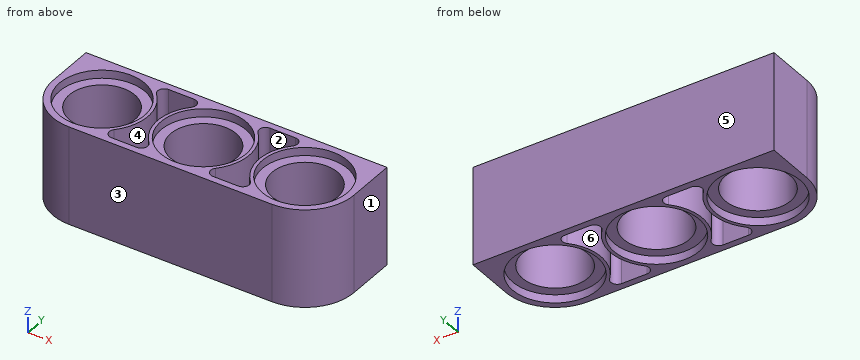
```python
from build123d import *

# Parameters (mm, degrees)
SKETCH1_R           = 3.302
SKETCH1_R_2         = 2.54
BOSS_EXTRUDE1_DEPTH = 3.81
SKETCH1_7_R         = 2.54
BOSS_EXTRUDE2_DEPTH = 3.81
SKETCH2_R           = 3.302
CUT_EXTRUDE1_DEPTH  = 0.635
BOSS_EXTRUDE3_DEPTH = 7.62


with BuildPart() as part:
    # Sketch1 → Boss-Extrude1 (new body)
    with BuildSketch(Plane.XY):
        with BuildLine():
            Line((3.937, -3.81), (7.874, -3.81))
            ThreePointArc((7.874, -3.81), (11.684, 0), (7.874, 3.81))
            Line((7.874, 3.81), (3.937, 3.81))
            Line((3.937, 3.81), (3.937, 3.302))
            Line((3.937, 3.302), (4.92278669, 3.302))
            ThreePointArc((4.92278669, 3.302), (5.389414486, 2.994804631), (5.291688354, 2.44475))
            ThreePointArc((5.291688354, 2.44475), (4.318, 0), (5.291688354, -2.44475))
            ThreePointArc((5.291688354, -2.44475), (5.389414486, -2.994804631), (4.92278669, -3.302))
            Line((4.92278669, -3.302), (3.937, -3.302))
            Line((3.937, -3.302), (3.937, -3.81))
        make_face()
        with Locations((7.874, 0)):
            Circle(SKETCH1_R, mode=Mode.SUBTRACT)
        with Locations((7.874, 0)):
            Circle(SKETCH1_R)
        with Locations(Location((7.874, 0, 0), (0, 0, 180))):
            Circle(SKETCH1_R_2, mode=Mode.SUBTRACT)
    extrude(amount=BOSS_EXTRUDE1_DEPTH)


with BuildPart() as body_2:
    # Sketch1_7 → Boss-Extrude2 (new body)
    with BuildSketch(Plane.XY):
        with BuildLine():
            Line((3.937, -3.81), (3.937, -3.302))
            Line((3.937, -3.302), (2.95121331, -3.302))
            ThreePointArc((2.95121331, -3.302), (2.484585514, -2.994804631), (2.582311646, -2.44475))
            ThreePointArc((2.582311646, -2.44475), (3.556, 0), (2.582311646, 2.44475))
            ThreePointArc((2.582311646, 2.44475), (2.484585514, 2.994804631), (2.95121331, 3.302))
            Line((2.95121331, 3.302), (3.937, 3.302))
            Line((3.937, 3.302), (3.937, 3.81))
            Line((3.937, 3.81), (-3.937, 3.81))
            Line((-3.937, 3.81), (-3.937, 3.302))
            Line((-3.937, 3.302), (-2.95121331, 3.302))
            ThreePointArc((-2.95121331, 3.302), (-2.484585514, 2.994804631), (-2.582311646, 2.44475))
            ThreePointArc((-2.582311646, 2.44475), (-3.556, 0), (-2.582311646, -2.44475))
            ThreePointArc((-2.582311646, -2.44475), (-2.484585514, -2.994804631), (-2.95121331, -3.302))
            Line((-2.95121331, -3.302), (-3.937, -3.302))
            Line((-3.937, -3.302), (-3.937, -3.81))
            Line((-3.937, -3.81), (3.937, -3.81))
        make_face()
        with Locations(Location((0, 0, 0), (0, 0, 180))):
            Circle(SKETCH1_7_R, mode=Mode.SUBTRACT)
    extrude(amount=BOSS_EXTRUDE2_DEPTH)


with BuildPart() as cut_extrude1_tool:
    # Sketch2 → Cut-Extrude1 (new body)
    with BuildSketch(Plane.XY):
        with Locations((7.874, 0)):
            Circle(SKETCH2_R)
        Circle(SKETCH2_R)
    extrude(amount=CUT_EXTRUDE1_DEPTH)


with BuildPart() as part_1:
    add(part.part)

    # Cut-Extrude1: cut by cut_extrude1_tool
    add(cut_extrude1_tool.part, mode=Mode.SUBTRACT)


with BuildPart() as body_2_1:
    add(body_2.part)

    # Cut-Extrude1: cut by cut_extrude1_tool
    add(cut_extrude1_tool.part, mode=Mode.SUBTRACT)


with BuildPart() as body_3:
    # Mirror2: mirrored copy
    add(part_1.part.mirror(Plane(origin=(0, 0, 0), x_dir=(0, 0, 1), z_dir=(1, 0, 0))))


with BuildPart() as part_2:
    add(part_1.part)

    # Combine1: union body 3, body 2
    add(body_3.part)
    add(body_2_1.part)

    # Mirror3: part across plane


with BuildPart() as part_3:
    add(part_2.part)
    add(part_2.part.mirror(Plane.XY.offset(3.81)))

    # Sketch3 → Boss-Extrude3 (add, through all)
    with BuildSketch(Plane.XY.offset(7.62)):
        with BuildLine():
            Line((7.874, 3.81), (11.684, 3.81))
            Line((11.684, 3.81), (11.684, 0))
            ThreePointArc((11.684, 0), (10.568076836, 2.694076836), (7.874, 3.81))
        make_face()
    boss_extrude3 = extrude(amount=-BOSS_EXTRUDE3_DEPTH)

    # Mirror4: Boss-Extrude3 across plane
    add(boss_extrude3.mirror(Plane(origin=(0, 0, 0), x_dir=(0, 0, 1), z_dir=(1, 0, 0))))


solid = part_3.part
```
Check sheet for the modelled part. Datum: model origin and axes. Units: mm. Face numbers are marked on the shaded views. A direction names the side the tool comes from. Coordinates: 2 decimals unless noted, no trailing zeros. Write each loop counter-clockwise with the first axis right and the second up, starting at its lowest first coordinate (ties: lowest second). Pieces come first, ordered by that corner, then holes. Notation, with made-up numbers: (83, -26.5) - (138, -26.5) arc R26 cw to (138, -10.5) - close; hole circle Ø8 at (78.25, 69.5). An arc over 180 degrees is marked (long way). One line per question, with ' | ' between items.
Item 1: Mould release check, pull along X, two halves, no side actions. Record for the marked faces 1, 2, 3 and 4: pulls with the +X half, pulls with the -X half, needs draft (parallel to the pull), parting line crosses it, or undercut.
Determined:
face 1: pulls with the +X half | face 2: undercut | face 3: needs draft | face 4: undercut
Item 2: Sectioned sample at A-A on z = 2.5. Record the boundary of the cut face in (x, y), plus the area to 3 significant figures.
Determined:
outline: (-11.68, 0) arc R3.81 ccw to (-7.87, -3.81) - (7.87, -3.81) arc R3.81 ccw to (11.68, 0) - (11.68, 3.81) - (-11.68, 3.81) - close; hole circle Ø5.08 at (-7.87, 0); hole (-5.29, -2.44) arc R0.51 ccw to (-4.92, -3.3) - (-2.95, -3.3) arc R0.51 ccw to (-2.58, -2.44) arc R3.56 cw to (-2.58, 2.44) arc R0.51 ccw to (-2.95, 3.3) - (-4.92, 3.3) arc R0.51 ccw to (-5.29, 2.44) arc R3.56 cw to start; hole circle Ø5.08 at (0, 0); hole (2.58, -2.44) arc R0.51 ccw to (2.95, -3.3) - (4.92, -3.3) arc R0.51 ccw to (5.29, -2.44) arc R3.56 cw to (5.29, 2.44) arc R0.51 ccw to (4.92, 3.3) - (2.95, 3.3) arc R0.51 ccw to (2.58, 2.44) arc R3.56 cw to start; hole circle Ø5.08 at (7.87, 0) | area: 87.9 mm2
Item 3: Sectioned sample at B-B on x = 0. Record the boundary of the cut face in (y, z) (3 decimals), plus the area to 3 significant figures.
Determined:
outline: (-3.81, 0) - (-3.302, 0) - (-3.302, 0.635) - (-2.54, 0.635) - (-2.54, 6.985) - (-3.302, 6.985) - (-3.302, 7.62) - (-3.81, 7.62) - close; (2.54, 0.635) - (3.302, 0.635) - (3.302, 0) - (3.81, 0) - (3.81, 7.62) - (3.302, 7.62) - (3.302, 6.985) - (2.54, 6.985) - close | area: 17.4 mm2
Item 4: Thickness scan on line 1 (X direction, y = -2.75, z = 1); line 2 (Y direction, x = 0, z = 0.35); line 3 (X direction, y = 0.25, z = 1.25). Record the ranges inside material, lowest first. Write a range as [from, to].
Determined:
line 1: x = [-10.51, -5.43], [-2.45, 2.45], [5.43, 10.51] | line 2: y = [-3.81, -3.3], [3.3, 3.81] | line 3: x = [-11.68, -10.4], [-5.35, -4.33], [-3.55, -2.53], [2.53, 3.55], [4.33, 5.35], [10.4, 11.68]
Item 5: Gauge pin test, flat ends, axial feed: P1, Ø3.5, axis at x = -8, y = 1, coming from the -Z side (3 decimals); P2, Ø1, axis at x = -9.5, y = 2, coming from the +Z side (3 decimals). Record the tip position at first contact, or that the pin passes through.
Determined:
P1: stops at z = 0.635 | P2: stops at z = 6.985
Item 6: Sectioned sample at C-C on y = -2.75. Give the number of separate pieces and of enclosed holes in the cut face, plus the area to 3 significant figures.
Determined:
separate pieces: 3 | enclosed holes: 0 | area: 101 mm2
Item 7: Access from +Z, -Z, +X, -X, +Y, -Y to the whole of each face (thin tool, end or side, straight path). Record for the marked faces 5 and 6.
Determined:
face 5: +Z, -Z, +X, -X, +Y | face 6: +Z, -Z
